Source: three-view drawing plus pictorial views. Frame: mm from the lowest corner of the part. A direction names the side the tool comes from. Coordinates: 2 decimals unless noted, no trailing zeros. Loops run counter-clockwise (first coordinate to the right, second up) from the corner with the lowest first, then second, coordinate; pieces in that order, holes last. Notation, with made-up numbers: (55, 34.25) - (114, 34.25) arc R19 cw to (114, 43.25) - close; hole circle Ø7 at (2, -19.5). An arc over 180 degrees is marked (long way). Return JSON: item names as keys, results as strings.
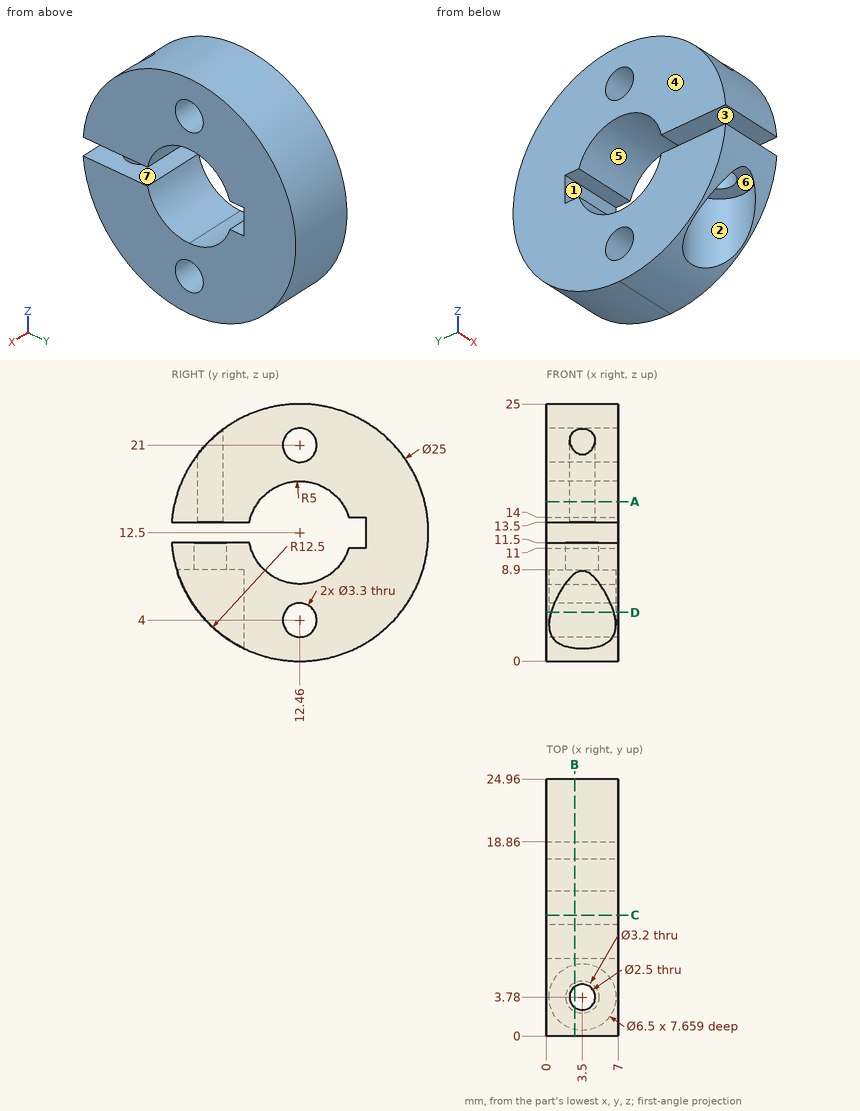
Item 1: Ray query, probe 1 along Y at (x, z) = (2.5, 20.5) (1 decimal); probe 2 along Y at (x, z) = (3.5, 10.7) (1 decimal); probe 3 along X at (y, z) = (4.75, 3.5). Return the intervals inside material, ascending. Write a range as from..to.
Worked out:
{"probe 1": "2.9..3, 4.5..10.9, 14..22.1", "probe 2": "0.1..2.2, 5.4..7.8, 17.1..24.8", "probe 3": "0..0.4, 6.6..7"}
Item 2: Mould query, pull axis Z, two halves, no side actions, for the marked faces 4, 5, 6 and 7. Classes: +Z half, -Z half, draft (parallel to the pull), parting line (faces both ways), or undercut.
Worked out:
{"face 4": "draft", "face 5": "undercut", "face 6": "-Z half", "face 7": "undercut"}
Item 3: Section query C-C, the plane y = 11.75. Return loops of the section in (x, z).
Worked out:
{"outline": "(0, 0.02) - (7, 0.02) - (7, 2.51) - (0, 2.51) - close; (0, 5.49) - (7, 5.49) - (7, 7.55) - (0, 7.55) - close; (0, 17.45) - (7, 17.45) - (7, 19.51) - (0, 19.51) - close; (0, 22.49) - (7, 22.49) - (7, 24.98) - (0, 24.98) - close"}
Item 4: Reachability of the marked faces 1, 2 and 3 from +Z, -Z, +X, -X, +Y, -Y: full face, straight path, thin tool, end or side. Return the list, or none.
Worked out:
{"face 1": "+X, -X", "face 2": "-Z", "face 3": "+X, -X, -Y"}
Item 5: Section query A-A, the plane z = 15.5. Count the separate pieces of the cut face and the enclosed holes in it, and give its area (3 significant figures).
Worked out:
{"separate pieces": "2", "enclosed holes": "1", "area": "109 mm^2"}
Item 6: Section query D-D, the plane z = 4.75. Return loops of the section in (x, y).
Worked out:
{"outline": "(0, 2.65) - (0.45, 2.65) arc R3.25 cw (long way) to (6.55, 2.65) - (7, 2.65) - (7, 10.99) - (0, 10.99) - close; (0, 13.93) - (7, 13.93) - (7, 22.27) - (0, 22.27) - close"}
Item 7: First-contact query: pin 1 Ø4 at (x, y) = (3.5, 3.78) entering from -Z; pin 2 Ø1.3 at (x, y) = (4.5, 18) entering from +Z; pin 3 Ø1.5 at (x, z) = (3, 18) entering from -Y; pin 4 Ø3.5 at (x, z) = (2.5, 12) entering from -Y. Flat tips, straight axial feed; report the tip coordinate or a pass-through.
Worked out:
{"pin 1": "z = 8.9", "pin 2": "z = 24", "pin 3": "y = 0.9", "pin 4": "y = 0"}
Item 8: Section query B-B, the plane x = 2.75. Return loops of the section in (y, z), and give its area (3 significant figures).
Worked out:
{"outline": "(0, 11.5) arc R12.5 ccw to (0.62, 8.5) - (0.62, 8.9) - (2.37, 8.9) - (2.37, 11.5) - close; (0, 13.5) - (2.78, 13.5) - (2.78, 20.41) arc R12.5 ccw to start; (4.78, 13.5) - (7.56, 13.5) arc R5 cw to (17.23, 14) - (18.86, 14) - (18.86, 11) - (17.23, 11) arc R5 cw to (7.56, 11.5) - (5.19, 11.5) - (5.19, 8.9) - (6.94, 8.9) - (6.94, 1.28) arc R12.5 ccw (long way) to (4.78, 22.36) - close; hole circle Ø3.3 at (12.46, 4); hole circle Ø3.3 at (12.46, 21)", "area": "321 mm^2"}
